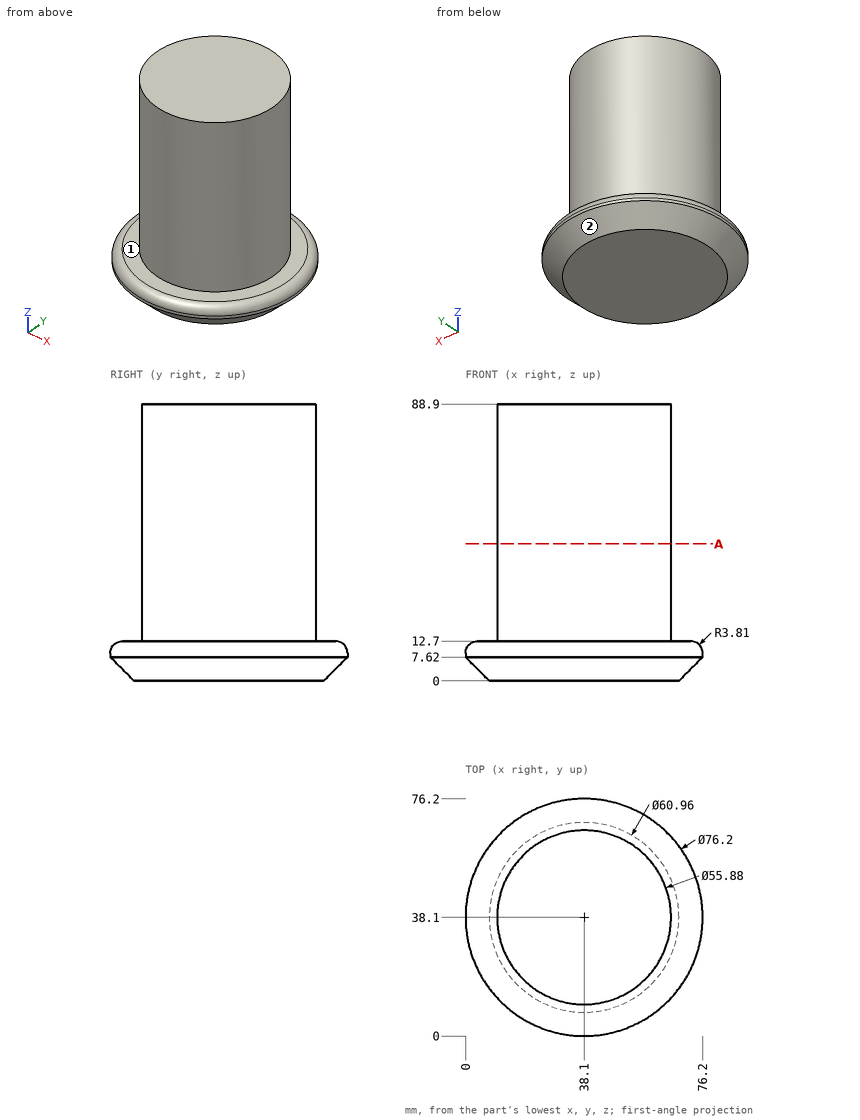
Geometry check sheet. Reference: drawing and pictorial views, mm from the part's lowest x, y, z. A direction names the side the tool comes from. Give positions to 0.01 mm unless a question says otherwise; leave off trailing zeros. Order: outer loops, then holes, each group sorted by start corner. A loop starts at its lowest first (then second) coordinate and runs counter-clockwise, first axis right, second up. Notation, with made-up numbers: M 71,26 L 101,26 A15 ccw 101,54 Z; hole C -22.75,81 d10. An arc over 180 degrees is marked long. Answer in a Markdown table with one row per item.
1) Gauge pin test, flat ends, axial feed: P1, Ø1.5, axis at x = 32.5, z = 47.5, coming from the -Y side; P2, Ø5, axis at x = 37, z = 64.5, coming from the +Y side; P3, Ø1.5, axis at x = 64, y = 12, coming from the +Z side. Record the tip position at first contact, or that the pin passes through.
Filled sheet:
| item | result |
|---|---|
| P1 | stops at y = 10.58 |
| P2 | stops at y = 66.04 |
| P3 | stops at z = 12.28 |
2) Access from +Z, -Z, +X, -X, +Y, -Y to the whole of each face (thin tool, end or side, straight path). Record for the marked faces 1 and 2.
Filled sheet:
| item | result |
|---|---|
| face 1 | +Z |
| face 2 | -Z |
3) Thickness scan on L1, parallel to Y at x = 50.5, z = 61; L2, parallel to X at y = 22.5, z = 62.5; L3, parallel to Y at x = 53, z = 72. Record the ranges inside material, lowest first. Write a range as [from, to].
Filled sheet:
| item | result |
|---|---|
| L1 | y = [13.06, 63.14] |
| L2 | x = [14.92, 61.28] |
| L3 | y = [14.46, 61.74] |
4) Cross-section at A-A, the plane z = 44. Enter the section's corners in (x, y).
Filled sheet:
| item | result |
|---|---|
| outline | C 38.1,38.1 d55.88 |
